from build123d import *

# Parameters (mm, degrees)
SKETCH1_R          = 2.25
BASE_FLANGE1_DEPTH = 4
CUT_EXTRUDE1_REACH = 101.076
SKETCH5_R          = 2.25
CUT_EXTRUDE2_DEPTH = 100.075728612
SKETCH6_R          = 2.25
CUT_EXTRUDE3_DEPTH = 100.075728612
SKETCH8_W          = 5
SKETCH8_H          = 102.679491924
SKETCH8_W_2        = 102.679491924
SKETCH8_H_2        = 5
TAB1_DEPTH         = 4
SKETCH7_R          = 2.25
CUT_EXTRUDE4_DEPTH = 100.075728612
SKETCH9_R          = 2.25
CUT_EXTRUDE5_DEPTH = 100.075728612


# Sheet-metal steps are written as plain solids
with BuildPart() as part:
    # Sketch1 → Base-Flange1 (new body)
    with BuildSketch(Plane(origin=(0, 0, 0), x_dir=(1, 0, 0), z_dir=(0, 1, 0))):
        with BuildLine():
            Line((-60, 0), (-60, 42.679491924))
            ThreePointArc((-60, 42.679491924), (-61.339745962, 47.679491924), (-65, 51.339745962))
            ThreePointArc((-65, 51.339745962), (-67.071067812, 67.071067812), (-51.339745962, 65))
            ThreePointArc((-51.339745962, 65), (-47.679491924, 61.339745962), (-42.679491924, 60))
            Line((-42.679491924, 60), (0, 60))
            Line((0, 60), (42.679491924, 60))
            ThreePointArc((42.679491924, 60), (47.679491924, 61.339745962), (51.339745962, 65))
            ThreePointArc((51.339745962, 65), (67.071067812, 67.071067812), (65, 51.339745962))
            ThreePointArc((65, 51.339745962), (61.339745962, 47.679491924), (60, 42.679491924))
            Line((60, 42.679491924), (60, 0))
            Line((60, 0), (60, -42.679491924))
            ThreePointArc((60, -42.679491924), (61.339745962, -47.679491924), (65, -51.339745962))
            ThreePointArc((65, -51.339745962), (67.071067812, -67.071067812), (51.339745962, -65))
            ThreePointArc((51.339745962, -65), (47.679491924, -61.339745962), (42.679491924, -60))
            Line((42.679491924, -60), (0, -60))
            Line((0, -60), (-42.679491924, -60))
            ThreePointArc((-42.679491924, -60), (-47.679491924, -61.339745962), (-51.339745962, -65))
            ThreePointArc((-51.339745962, -65), (-67.071067812, -67.071067812), (-65, -51.339745962))
            ThreePointArc((-65, -51.339745962), (-61.339745962, -47.679491924), (-60, -42.679491924))
            Line((-60, -42.679491924), (-60, 0))
        make_face()
        with Locations(Location((-60, 60, 0), (0, 0, 270))):
            Circle(SKETCH1_R, mode=Mode.SUBTRACT)
        with Locations(Location((60, 60, 0), (0, 0, 270))):
            Circle(SKETCH1_R, mode=Mode.SUBTRACT)
        with Locations(Location((60, -60, 0), (0, 0, 270))):
            Circle(SKETCH1_R, mode=Mode.SUBTRACT)
        with Locations(Location((-60, -60, 0), (0, 0, 270))):
            Circle(SKETCH1_R, mode=Mode.SUBTRACT)
    extrude(amount=-BASE_FLANGE1_DEPTH)

    # Sketch4 → Cut-Extrude1 (cut, up to next)
    with BuildSketch(Plane(origin=(0, 0, 0), x_dir=(1, 0, 0), z_dir=(0, 1, 0)), mode=Mode.PRIVATE) as cut_extrude1_sk1:
        Polygon((-20.5, 22.5), (20.5, 22.5), (22.5, 20.5), (22.5, -20.5), (20.5, -22.5), (-20.5, -22.5), (-22.5, -20.5), (-22.5, 20.5), align=None)
    cut_extrude1_tool1 = extrude(cut_extrude1_sk1.sketch, amount=-CUT_EXTRUDE1_REACH, mode=Mode.PRIVATE) & part.part
    add(cut_extrude1_tool1.solids().sort_by_distance((0, 0, 0))[0], mode=Mode.SUBTRACT)

    # Sketch5 → Cut-Extrude2 (cut, through all)
    with BuildSketch(Plane.XZ.offset(4)):
        with Locations(Location((-54.343145751, 54.343145751, 0), (0, 0, 270))):
            Circle(SKETCH5_R)
        with Locations(Location((54.343145751, 54.343145751, 0), (0, 0, 270))):
            Circle(SKETCH5_R)
        with Locations(Location((54.343145751, -54.343145751, 0), (0, 0, 270))):
            Circle(SKETCH5_R)
        with Locations(Location((-54.343145751, -54.343145751, 0), (0, 0, 270))):
            Circle(SKETCH5_R)
    extrude(amount=-CUT_EXTRUDE2_DEPTH, mode=Mode.SUBTRACT)

    # Sketch6 → Cut-Extrude3 (cut, through all)
    with BuildSketch(Plane.XZ.offset(4)):
        with Locations(Location((27.5, 15, 0), (0, 0, 270))):
            Circle(SKETCH6_R)
        with Locations(Location((27.5, -15, 0), (0, 0, 270))):
            Circle(SKETCH6_R)
        with Locations(Location((-27.5, -15, 0), (0, 0, 270))):
            Circle(SKETCH6_R)
        with Locations(Location((-27.5, 15, 0), (0, 0, 270))):
            Circle(SKETCH6_R)
    extrude(amount=-CUT_EXTRUDE3_DEPTH, mode=Mode.SUBTRACT)

    # Sketch8 → Tab1 (add)
    with BuildSketch(Plane.XZ.offset(4)):
        with Locations((-62.5, 0)):
            Rectangle(SKETCH8_W, SKETCH8_H)
        with Locations((0, -62.5)):
            Rectangle(SKETCH8_W_2, SKETCH8_H_2)
        with Locations((62.5, 0)):
            Rectangle(SKETCH8_W, SKETCH8_H)
        with Locations((0, 62.5)):
            Rectangle(SKETCH8_W_2, SKETCH8_H_2)
    extrude(amount=-TAB1_DEPTH)

    # Sketch7 → Cut-Extrude4 (cut, through all)
    with BuildSketch(Plane.XZ.offset(4)):
        with Locations(Location((-16, 46, 0), (0, 0, 270))):
            Circle(SKETCH7_R)
        with Locations(Location((-16, 30, 0), (0, 0, 270))):
            Circle(SKETCH7_R)
        with Locations(Location((16, 30, 0), (0, 0, 90))):
            Circle(SKETCH7_R)
        with Locations(Location((16, 46, 0), (0, 0, 90))):
            Circle(SKETCH7_R)
        with Locations(Location((16, -46, 0), (0, 0, 270))):
            Circle(SKETCH7_R)
        with Locations(Location((16, -30, 0), (0, 0, 270))):
            Circle(SKETCH7_R)
        with Locations(Location((-16, -30, 0), (0, 0, 90))):
            Circle(SKETCH7_R)
        with Locations(Location((-16, -46, 0), (0, 0, 90))):
            Circle(SKETCH7_R)
    extrude(amount=-CUT_EXTRUDE4_DEPTH, mode=Mode.SUBTRACT)

    # Sketch9 → Cut-Extrude5 (cut, through all)
    with BuildSketch(Plane.XZ.offset(4)):
        with Locations(Location((-34.5, 56.5, 0), (0, 0, 270))):
            Circle(SKETCH9_R)
        with Locations(Location((-34.5, 41.5, 0), (0, 0, 270))):
            Circle(SKETCH9_R)
        with Locations(Location((-56.5, 0, 0), (0, 0, 270))):
            Circle(SKETCH9_R)
        with Locations(Location((-41.5, 0, 0), (0, 0, 270))):
            Circle(SKETCH9_R)
        with Locations(Location((-34.5, -41.5, 0), (0, 0, 270))):
            Circle(SKETCH9_R)
        with Locations(Location((-34.5, -56.5, 0), (0, 0, 270))):
            Circle(SKETCH9_R)
        with Locations(Location((34.5, -56.5, 0), (0, 0, 90))):
            Circle(SKETCH9_R)
        with Locations(Location((34.5, -41.5, 0), (0, 0, 90))):
            Circle(SKETCH9_R)
        with Locations(Location((41.5, 0, 0), (0, 0, 90))):
            Circle(SKETCH9_R)
        with Locations(Location((56.5, 0, 0), (0, 0, 90))):
            Circle(SKETCH9_R)
        with Locations(Location((34.5, 41.5, 0), (0, 0, 90))):
            Circle(SKETCH9_R)
        with Locations(Location((34.5, 56.5, 0), (0, 0, 90))):
            Circle(SKETCH9_R)
    extrude(amount=-CUT_EXTRUDE5_DEPTH, mode=Mode.SUBTRACT)


solid = part.part
Source: CAD feature listing. Evaluate the final solid. Frame: model axes, mm. A direction names the side the tool comes from. Give positions to 0.01 mm unless a question says otherwise; leave off trailing zeros. Write each loop counter-clockwise with the first axis right and the second up, starting at its lowest first coordinate (ties: lowest second). Pieces come first, ordered by that corner, then holes. Notation, with made-up numbers: (78, -19.75) - (109, -19.75) arc R36 ccw to (109, 14.25) - close; hole circle Ø5 at (39.25, 57). An arc over 180 degrees is marked (long way). Write item = value, one per line. Start each with the question number.
Q1. Cut plane A-A, the plane x = 16. Return loops of the section in (y, z).
Q2. Cut plane C-C, the plane x = -4.5. Return loops of the section in (y, z), then the cut area to 3 significant figures.
Q3. Cut plane B-B, the plane z = 41.5. Return loops of the section in (x, y), then the cut area to 3 significant figures.
Q4. Cut plane D-D, the plane y = -2.55. Give the number of separate pieces and of enclosed holes in the cut face, then the cut area to 3 significant figures.
Q5. Pin query (flat end, axial travel): pin 1 Ø5 at (x, z) = (-16, 30) entering from -Y; pin 2 Ø3.5 at (x, z) = (60, 60) entering from +Y; pin 3 Ø2 at (y, z) = (-2.5, 6.5) entering from +X; pin 4 Ø2 at (y, z) = (-2, 1) entering from -X. Return the tip coordinate at first contact, or that it passes through.
Q6. Reachability of faces 3 (the flat face through (65, -2, -1)), 4 (the flat face through (-22.5, -2, 0)) from +Z, -Z, +X, -X, +Y, -Y: full face, straight path, thin tool, end or side. Return the list, or none.
Q7. Material intervals for probe 1 along X at (y, z) = (-2.3, -46); probe 2 along Z at (x, y) = (34.5, -2.55); probe 3 along X at (y, z) = (-1.05, -14), sorted ascending.
Q8. Draft query along Z for faces 1 (the flat face through (-1, -2, 65)), 2 (the cylindrical face through (-29.496, -2.028, -16.038)). Return one class per face: +Z half, -Z half, draft (parallel to the pull), parting line (faces both ways), or undercut.
Computed values:
q1.outline = (-4, -65) - (0, -65) - (0, -48.25) - (-4, -48.25) - close; (-4, -43.75) - (0, -43.75) - (0, -32.25) - (-4, -32.25) - close; (-4, -27.75) - (0, -27.75) - (0, -22.5) - (-4, -22.5) - close; (-4, 22.5) - (0, 22.5) - (0, 27.75) - (-4, 27.75) - close; (-4, 32.25) - (0, 32.25) - (0, 43.75) - (-4, 43.75) - close; (-4, 48.25) - (0, 48.25) - (0, 65) - (-4, 65) - close
q2.outline = (-4, -65) - (0, -65) - (0, -22.5) - (-4, -22.5) - close; (-4, 22.5) - (0, 22.5) - (0, 65) - (-4, 65) - close
q2.area = 340 mm²
q3.outline = (-65, -4) - (-36.75, -4) - (-36.75, 0) - (-65, 0) - close; (-32.25, -4) - (32.25, -4) - (32.25, 0) - (-32.25, 0) - close; (36.75, -4) - (65, -4) - (65, 0) - (36.75, 0) - close
q3.area = 484 mm²
q4.separate_pieces = 1
q4.enclosed_holes = 33
q4.area = 14,800 mm²
q5.pin_1 = -4
q5.pin_2 = through
q5.pin_3 = 65
q5.pin_4 = -65
q6.face_3 = +X, +Y, -Y
q6.face_4 = +Y, -Y
q7.probe_1 = -65 to -18.25, -13.75 to 13.75, 18.25 to 65
q7.probe_2 = -65 to -58.75, -54.25 to -43.75, -39.25 to 39.25, 43.75 to 54.25, 58.75 to 65
q7.probe_3 = -65 to -29.52, -25.48 to -22.5, 22.5 to 25.48, 29.52 to 65
q8.face_1 = +Z half
q8.face_2 = undercut
